```python
from build123d import *

# Parameters (mm, degrees)
F0_R     = 4.6
F1_DEPTH = 4


with BuildPart() as f1:
    # F0 (on Front) → F1 (new body)
    with BuildSketch(Plane.XZ):
        with BuildLine():
            Line((-46.75, 31.8), (-46.75, 0))
            ThreePointArc((-46.75, 0), (-40.283024, -12.33643), (-26.458333, -14.035607))
            ThreePointArc((-26.458333, -14.035607), (-15.875, -12.106821), (-5.291667, -14.035607))
            ThreePointArc((-5.291667, -14.035607), (8.533024, -12.33643), (15, 0))
            Line((15, 0), (15, 31.8))
            Line((15, 31.8), (15, 44))
            Line((15, 44), (-46.75, 44))
            Line((-46.75, 44), (-46.75, 31.8))
        make_face()
        with BuildLine():
            ThreePointArc((-36.515, 0), (-31.75, 4.765), (-26.985, 0))
            ThreePointArc((-26.985, 0), (-31.75, -4.765), (-36.515, 0))
        make_face(mode=Mode.SUBTRACT)
        with BuildLine():
            ThreePointArc((-4.765, 0), (0, 4.765), (4.765, 0))
            ThreePointArc((4.765, 0), (0, -4.765), (-4.765, 0))
        make_face(mode=Mode.SUBTRACT)
        with Locations((-15.875, 31.8)):
            Circle(F0_R, mode=Mode.SUBTRACT)
    extrude(amount=-F1_DEPTH)


solid = f1.part
```
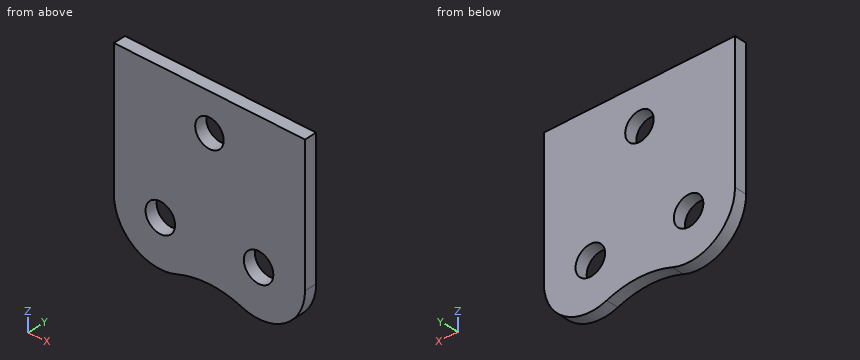
Geometry: final body of the model. Coordinates: model frame, mm. Coordinates: 2 decimals unless noted, no trailing zeros. Order: outer loops, then holes, each group sorted by start corner. A loop starts at its lowest first (then second) coordinate and runs counter-clockwise, first axis right, second up.
Item 1: Section query B-B (y = 2.6). Output: boundary loops of the cut face in (x, z) (3 decimals).
Answer:
outline: (-46.75, 0) arc R15 ccw to (-26.458, -14.036) arc R30 cw to (-5.292, -14.036) arc R15 ccw to (15, 0) - (15, 44) - (-46.75, 44) - close; hole circle Ø9.53 at (-31.75, 0); hole circle Ø9.2 at (-15.875, 31.8); hole circle Ø9.53 at (0, 0)
Item 2: Section query D-D (x = -1). Output: boundary loops of the cut face in (y, z).
Answer:
outline: (0, -14.97) - (4, -14.97) - (4, -4.66) - (0, -4.66) - close; (0, 4.66) - (4, 4.66) - (4, 44) - (0, 44) - close
Item 3: Contact query for flat-ended pins moving along their axis: P1, Ø2, axis at x = -33, y = 2, coming from the -Z side; P2, Ø5.5, axis at x = -31.75, z = 0, coming from the +Y side; P3, Ø1.5, axis at y = 1, z = -5, coming from the +X side. Output: stop coordinate, or through.
Answer:
P1: stops at z = -15
P2: passes through
P3: stops at x = 14.39
Item 4: Material intervals for line 1 along Z through (x, y) = (-31.75, 1.35) (3 decimals); line 2 along Z through (x, y) = (-15.5, 1.2); line 3 along X through (y, z) = (0.3, 31), sorted ascending.
Answer:
line 1: z = -15 to -4.765, 4.765 to 44
line 2: z = -12.11 to 27.22, 36.38 to 44
line 3: x = -46.75 to -20.4, -11.35 to 15
Item 5: Section query A-A (x = -31.75). Output: boundary loops of the cut face in (y, z) (3 decimals).
Answer:
outline: (0, -15) - (4, -15) - (4, -4.765) - (0, -4.765) - close; (0, 4.765) - (4, 4.765) - (4, 44) - (0, 44) - close
Item 6: Section query C-C (z = 3). Output: boundary loops of the cut face in (x, y).
Answer:
outline: (-46.75, 0) - (-35.45, 0) - (-35.45, 4) - (-46.75, 4) - close; (-28.05, 0) - (-3.7, 0) - (-3.7, 4) - (-28.05, 4) - close; (3.7, 0) - (15, 0) - (15, 4) - (3.7, 4) - close
